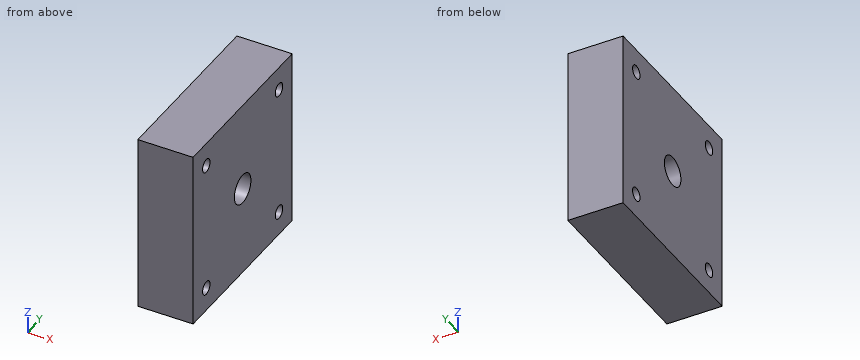
Autodesk Inventor part; units mm, degrees
ref_plane "YZ Plane" through (0, 0, 0) normal (1, 0, 0) x (0, 1, 0)
ref_plane "XZ Plane" through (0, 0, 0) normal (0, 1, 0) x (-1, 0, 0)
ref_plane "XY Plane" through (0, 0, 0) normal (0, 0, 1) x (1, 0, 0)
sketch "Esquisse1" plane through (0, 0, 0) normal (1, 0, 0) x (0, 1, 0)
  line L0 (-30, -30) -> (30, -30)
  line L1 (30, -30) -> (30, 30)
  line L2 (30, 30) -> (-30, 30)
  line L3 (-30, 30) -> (-30, -30)
  line L4 (-30, -30) -> (30, 30) construction
  line L5 (30, -30) -> (-30, 30) construction
  circle A0 centre (22, 22) radius 2.25
  circle A1 centre (-22, 22) radius 2.25
  circle A2 centre (22, -22) radius 2.25
  circle A3 centre (-22, -22) radius 2.25
  point P0 (0, 0)
  dimension "d0" = 60
  dimension "d1" = 8
  dimension "d2" = 4.5
extrude "Extrusion1" add sketch "Esquisse1" along normal blind 18.55
sketch "Esquisse2" plane through (18.55, 0, 0) normal (1, 0, 0) x (0, 0, -1)
  circle A0 centre (0, 0) radius 5
  dimension "d5" = 10
extrude "Extrusion2" cut sketch "Esquisse2" against normal blind 18.55
properties part number "nut_blocker"
CAD build for the part. Positions are in the model's coordinates, mm. Round coordinates to 2 decimals unless told otherwise and drop trailing zeros. Order: outer loops, then holes, each group sorted by start corner. A loop starts at its lowest first (then second) coordinate and runs counter-clockwise, first axis right, second up. Notation, with made-up numbers: (85, 61) -> (136, 61) arc R19 cw to (136, 80) -> close; hole circle Ø3 at (68, 12.5). An arc over 180 degrees is marked (long way). One line per question, with ' | ' between items.
Q1. Slice it at B-B (z = 22). Write the cut outline in (x, y), then the cut area to 3 significant figures.
Completed:
outline: (0, -30) -> (18.55, -30) -> (18.55, -24.25) -> (0, -24.25) -> close; (0, -19.75) -> (18.55, -19.75) -> (18.55, 19.75) -> (0, 19.75) -> close; (0, 24.25) -> (18.55, 24.25) -> (18.55, 30) -> (0, 30) -> close | area: 946 mm^2
Q2. Probe probe 1 along Z at (x, y) = (5.5, 22); probe 2 along Y at (x, z) = (12.75, 20); probe 3 along Y at (x, z) = (9.75, 0). List the from-to ranges inside material, lowest first.
Completed:
probe 1: z = -30 to -24.25, -19.75 to 19.75, 24.25 to 30 | probe 2: y = -30 to -23.03, -20.97 to 20.97, 23.03 to 30 | probe 3: y = -30 to -5, 5 to 30
Q3. Slice it at A-A (y = 0). Write the cut outline in (x, z).
Completed:
outline: (0, -30) -> (18.55, -30) -> (18.55, -5) -> (0, -5) -> close; (0, 5) -> (18.55, 5) -> (18.55, 30) -> (0, 30) -> close
Q4. Slice it at C-C (x = 10.25). Write the cut outline in (y, z), then the cut area to 3 significant figures.
Completed:
outline: (-30, -30) -> (30, -30) -> (30, 30) -> (-30, 30) -> close; hole circle Ø4.5 at (-22, -22); hole circle Ø4.5 at (-22, 22); hole circle Ø10 at (0, 0); hole circle Ø4.5 at (22, -22); hole circle Ø4.5 at (22, 22) | area: 3,460 mm^2
